CAD build for the part. Positions are in the model's coordinates, mm. Face numbers are marked on the shaded views. A direction names the side the tool comes from. Coordinates: 2 decimals unless noted, no trailing zeros. Write each loop counter-clockwise with the first axis right and the second up, starting at its lowest first coordinate (ties: lowest second). Pieces come first, ordered by that corner, then holes.
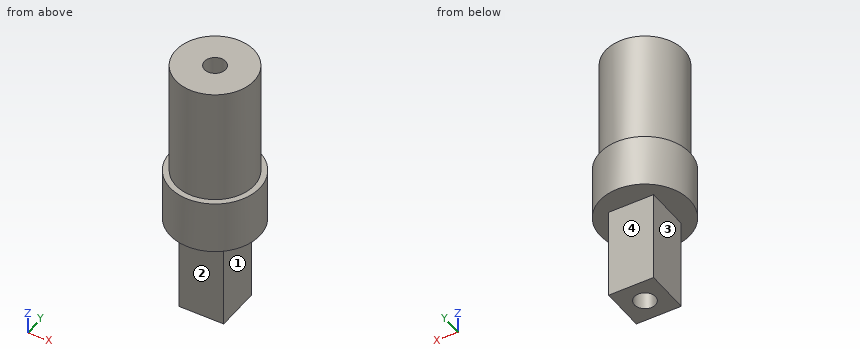
Autodesk Inventor part; units mm, degrees
ref_plane "XZ Plane" through (0, 0, 0) normal (0, 1, 0) x (-1, 0, 0)
ref_plane "XY Plane" through (0, 0, 0) normal (0, 0, 1) x (1, 0, 0)
sketch "Skizze1" plane through (0, 0, 0) normal (0, 0, 1) x (1, 0, 0)
  circle A0 centre (0, 0) radius 7.4
  dimension "d0" = 14.8
extrude "Extrusion1" add sketch "Skizze1" along normal mid plane 22
sketch "Skizze2" plane through (0, 0, -11) normal (0, 0, -1) x (-1, 0, 0)
  circle A0 centre (0, 0) radius 8.5
  dimension "d3" = 17
extrude "Extrusion2" add sketch "Skizze2" along normal blind 10
sketch "Skizze3" plane through (0, 0, -21) normal (0, 0, -1) x (-1, 0, 0)
  line L0 (-4.25, 4.25) -> (4.25, 4.25)
  line L1 (4.25, 4.25) -> (4.25, -4.25)
  line L2 (4.25, -4.25) -> (-4.25, -4.25)
  line L3 (-4.25, -4.25) -> (-4.25, 4.25)
  line L4 (-4.25, 4.25) -> (4.25, -4.25) construction
  line L5 (4.25, 4.25) -> (-4.25, -4.25) construction
  point P0 (0, 0)
  dimension "d6" = 8.5
  dimension "d7" = 8.5
extrude "Extrusion3" add sketch "Skizze3" along normal blind 17.4
sketch "Skizze4" plane through (0, 0, 11) normal (0, 0, 1) x (1, 0, 0)
  circle A0 centre (0, 0) radius 2
  dimension "d10" = 4
extrude "Extrusion4" cut sketch "Skizze4" against normal blind 5
sketch "Skizze5" plane through (0, 0, -38.4) normal (0, 0, -1) x (-1, 0, 0)
  circle A0 centre (0, 0) radius 2
  dimension "d13" = 4
extrude "Extrusion5" cut sketch "Skizze5" against normal blind 5
properties part number "_3D-Druck"
Item 1: Saw through at A-A, the plane y = 0. Write the cut outline in (x, z), and give its area (4 significant figures).
Item 2: Wall check: line 1 along Y through (x, z) = (0, -34.55); line 2 along Y through (x, z) = (0, 8.3); line 3 along Z through (x, y) = (-5, 6.5). Give the ranges that are in metal, low to high.
Item 3: Saw through at D-D, the plane x = -5. Write the cut outline in (y, z), and give its area (3 significant figures).
Item 4: Which spindle directions (+Z, -Z, +X, -X, +Y, -Y) get a long thin tool onto all of the face, cutting with end or side? Do the marked faces 1, 2, 3 and 4. Say none if no direction does.
Item 5: Flat gauge pins, fed straight in: pin 1 Ø5 at (y, z) = (-3.5, -33.5) entering from +X; pin 2 Ø8 at (y, z) = (-4, -31.5) entering from -X; pin 3 Ø2 at (x, z) = (1.5, -18) entering from -Y; pin 4 Ø5 at (x, y) = (1.5, -1) entering from -Z. Where does each tip first touch, or does it go through?
Item 6: Saw through at C-C, the plane z = -20.5. Write the cut outline in (x, y).
Working result:
1. outline: (-8.5, -21) - (-4.25, -21) - (-4.25, -38.4) - (-2, -38.4) - (-2, -33.4) - (2, -33.4) - (2, -38.4) - (4.25, -38.4) - (4.25, -21) - (8.5, -21) - (8.5, -11) - (7.4, -11) - (7.4, 11) - (2, 11) - (2, 6) - (-2, 6) - (-2, 11) - (-7.4, 11) - (-7.4, -11) - (-8.5, -11) - close
1. area: 603.5 mm2
2. line 1: y = -4.25 to -2, 2 to 4.25
2. line 2: y = -7.4 to -2, 2 to 7.4
2. line 3: z = -21 to -11
3. outline: (-6.87, -21) - (6.87, -21) - (6.87, -11) - (5.46, -11) - (5.46, 11) - (-5.46, 11) - (-5.46, -11) - (-6.87, -11) - close
3. area: 378 mm2
4. face 1: -Z, +X, +Y, -Y
4. face 2: -Z, +X, -X, -Y
4. face 3: -Z, -X, +Y, -Y
4. face 4: -Z, +X, -X, +Y
5. pin 1: stops at x = 4.25
5. pin 2: stops at x = -4.25
5. pin 3: stops at y = -8.49
5. pin 4: stops at z = -38.4
6. outline: circle Ø17 at (0, 0)
